Here's how the part is built. I have some questions about the finished solid (model axes, mm). A direction names the side the tool comes from. Give positions to 0.01 mm unless a question says otherwise; leave off trailing zeros. Order: outer loops, then holes, each group sorted by start corner. A loop starts at its lowest first (then second) coordinate and runs counter-clockwise, first axis right, second up.
from build123d import *

# Parameters (mm, degrees)
SKETCH1_W           = 42
SKETCH1_H           = 57
SKETCH1_R           = 2.5
BOSS_EXTRUDE1_DEPTH = 45
FILLET1_R           = 5
FILLET2_R           = 5
SKETCH2_R           = 10
SKETCH2_R_2         = 2.5
BOSS_EXTRUDE2_DEPTH = 1
FILLET3_R           = 1


# Some blends are built 0.0001 mm under size
with BuildPart() as part:
    # Sketch1 → Boss-Extrude1 (new body)
    with BuildSketch(Plane.XY):
        with Locations((-9, -11.5)):
            Rectangle(SKETCH1_W, SKETCH1_H)
        with Locations(Location((0, 0, 0), (0, 0, 180))):
            Circle(SKETCH1_R, mode=Mode.SUBTRACT)
    extrude(amount=BOSS_EXTRUDE1_DEPTH)

    # Fillet1
    fillet1_edges = [part.edges().sort_by_distance(p)[0] for p in [
        (12, -11.5, 45),
        (-9, 17, 45),
        (-30, -11.5, 45),
        (-9, 17, 0),
        (12, -11.5, 0),
        (-30, -11.5, 0),
        (-30, 17, 22.5),
        (12, 17, 22.5),
        (12, -40, 22.5),
        (-30, -40, 22.5),
        (-9, -40, 45),
    ]]
    fillet(fillet1_edges, radius=FILLET1_R)

    # Fillet2
    # the kernel refuses this fillet: 5 mm, written as the material it takes off along each edge
    with BuildSketch(Plane(origin=(7, -35, 5), x_dir=(0, -1, 0), z_dir=(0, 0, -1))) as fillet2_piece_1_section:
        Polygon((0, 0), (FILLET2_R, 0), (FILLET2_R, -FILLET2_R), (0, -FILLET2_R), align=None)
    fillet2_piece_1 = extrude(amount=FILLET2_R, mode=Mode.PRIVATE)
    fillet2_piece_1 = fillet2_piece_1 - Plane(origin=(7, -35, 5), x_dir=(-0.7071067811865477, 0.7071067811865474, 0), z_dir=(0, 0, -1)) * Sphere(FILLET2_R, mode=Mode.PRIVATE)
    add(fillet2_piece_1, mode=Mode.SUBTRACT)
    with BuildSketch(Plane(origin=(-25, -35, 5), x_dir=(0, -1, 0), z_dir=(0, 0, -1))) as fillet2_piece_2_section:
        Polygon((0, 0), (FILLET2_R, 0), (FILLET2_R, FILLET2_R), (0, FILLET2_R), align=None)
    fillet2_piece_2 = extrude(amount=FILLET2_R, mode=Mode.PRIVATE)
    fillet2_piece_2 = fillet2_piece_2 - Plane(origin=(-25, -35, 5), x_dir=(0.7071067811865474, 0.7071067811865476, 0), z_dir=(0, 0, -1)) * Sphere(FILLET2_R, mode=Mode.PRIVATE)
    add(fillet2_piece_2, mode=Mode.SUBTRACT)
    with BuildSketch(Plane(origin=(7, -40, 0), x_dir=(0, 1, 0), z_dir=(-1, 0, 0))) as fillet2_piece_3:
        with BuildLine():
            CenterArc((FILLET2_R, -FILLET2_R), FILLET2_R, 90, 90)
            Line((0, -FILLET2_R), (0, 0))
            Line((0, 0), (FILLET2_R, 0))
        make_face()
    extrude(amount=32, mode=Mode.SUBTRACT)

    # Sketch2 → Boss-Extrude2 (add)
    with BuildSketch(Plane.ZY.offset(30)):
        with Locations(Location((22.5, -11.5, 0), (0, 0, 180))):
            Circle(SKETCH2_R)
        with Locations((22.5, -11.5)):
            Circle(SKETCH2_R_2, mode=Mode.SUBTRACT)
    extrude(amount=BOSS_EXTRUDE2_DEPTH)

    # Fillet3
    fillet3_edges = [part.edges().sort_by_distance(p)[0] for p in [
        (-31, -11.5, 32.5),
    ]]
    fillet(fillet3_edges, radius=FILLET3_R - 0.0001)  # a hair under: the kernel refuses the full size


solid = part.part
Q1. Thinking about a two-plate mould opening in Y: for faces 1 (the face through (-29, -38, 23)), 2 (the face through (2.5, -0.1, 22.2)), 3 (the face through (-30, -12, 22)), 4 (the face through (-30, -22, 22)), which applies, released by +Y, released by -Y, zero draft, split by the parting line, or undercut?
Filled sheet:
face 1: released by -Y
face 2: undercut
face 3: undercut
face 4: zero draft
Q2. I need wall thicknesses on L1, parallel to Y at x = 0, z = 28; L2, parallel to X at y = -29.5, z = 36.5; L3, parallel to X at y = 1.5, z = 18.5. Which ranges of each line are inside material? Lowest first, please.
Filled sheet:
L1: y = -40 to -2.5, 2.5 to 17
L2: x = -30 to 12
L3: x = -30 to -2, 2 to 12
Q3. If we section it at C-C on x = 0: List the corners of the cut face in (y, z) for me.
Filled sheet:
outline: (-40, 5) arc R5 ccw to (-35, 0) - (-2.5, 0) - (-2.5, 45) - (-35, 45) arc R5 ccw to (-40, 40) - close; (2.5, 0) - (12, 0) arc R5 ccw to (17, 5) - (17, 40) arc R5 ccw to (12, 45) - (2.5, 45) - close
Q4. For faces 5 (the face through (-30.5, -13, 20.5)), 6 (the face through (-9, -38, 1)), which set-ups out of +Z, -Z, +X, -X, +Y, -Y let a thin tool reach every point of the face, with its end or its side?
Filled sheet:
face 5: -X
face 6: -Z, +X, -X, -Y
Q5. If we section it at B-B on z = 37: List the corners of the cut face in (x, y) for me, plus the area to 3 significant figures.
Filled sheet:
outline: (-30, -35) arc R5 ccw to (-25, -40) - (7, -40) arc R5 ccw to (12, -35) - (12, 12) arc R5 ccw to (7, 17) - (-25, 17) arc R5 ccw to (-30, 12) - close; hole circle Ø5 at (0, 0)
area: 2,350 mm2
Q6. If we section it at A-A on y = 0: List the corners of the cut face in (x, z) for me, plus the area to 3 significant figures.
Filled sheet:
outline: (-30, 5) arc R5 ccw to (-25, 0) - (-2.5, 0) - (-2.5, 45) - (-25, 45) arc R5 ccw to (-30, 40) - close; (2.5, 0) - (7, 0) arc R5 ccw to (12, 5) - (12, 40) arc R5 ccw to (7, 45) - (2.5, 45) - close
area: 1,640 mm2
Q7. I'm going to push flat-ended pins straight in: P1, Ø4, axis at y = -25.5, z = 10.5, coming from the -X side; P2, Ø4, axis at x = 0, y = 0, coming from the +Z side. Where does each tip first touch, or does it pass through?
Filled sheet:
P1: stops at x = -30
P2: passes through
